Geometry check sheet. Reference: the model listing, model coordinates, mm. A direction names the side the tool comes from. Coordinates: 2 decimals unless noted, no trailing zeros. Loops run counter-clockwise (first coordinate to the right, second up) from the corner with the lowest first, then second, coordinate; pieces in that order, holes last. Notation, with made-up numbers: (0.5, 23) -> (52.5, 23) arc R35 cw to (52.5, 57) -> close; hole circle Ø1 at (50.25, 62). An arc over 180 degrees is marked (long way). Answer as a JSON object with one key per item and string values.
from build123d import *

# Parameters (mm, degrees)
SKETCH_1_R      = 3.5
EXTRUDE_1_DEPTH = 3
FILLET_1_R      = 0.5


with BuildPart() as part:
    # Эскиз1 → Бобышка-Вытянуть1 (new body)
    with BuildSketch(Plane(origin=(0, 0, 0), x_dir=(1, 0, 0), z_dir=(0, 1, 0))):
        Polygon((-56.25, -20.75), (56.25, -20.75), (56.25, -15.25), (59.25, -15.25), (59.25, -5.25), (56.25, -5.25), (56.25, 0), (-56.25, 0), (-56.25, -5.25), (-59.25, -5.25), (-59.25, -15.25), (-56.25, -15.25), align=None)
        with Locations((-40.25, -13.1)):
            Circle(SKETCH_1_R, mode=Mode.SUBTRACT)
        with Locations((-31.305555556, -13.1)):
            Circle(SKETCH_1_R, mode=Mode.SUBTRACT)
        with Locations((-22.361111111, -13.1)):
            Circle(SKETCH_1_R, mode=Mode.SUBTRACT)
        with Locations((-13.416666667, -13.1)):
            Circle(SKETCH_1_R, mode=Mode.SUBTRACT)
        with Locations((-4.472222222, -13.1)):
            Circle(SKETCH_1_R, mode=Mode.SUBTRACT)
        with Locations((4.472222222, -13.1)):
            Circle(SKETCH_1_R, mode=Mode.SUBTRACT)
        with Locations((13.416666667, -13.1)):
            Circle(SKETCH_1_R, mode=Mode.SUBTRACT)
        with Locations((22.361111111, -13.1)):
            Circle(SKETCH_1_R, mode=Mode.SUBTRACT)
        with Locations((31.305555556, -13.1)):
            Circle(SKETCH_1_R, mode=Mode.SUBTRACT)
        with Locations((40.25, -13.1)):
            Circle(SKETCH_1_R, mode=Mode.SUBTRACT)
    extrude(amount=EXTRUDE_1_DEPTH)

    # Скругление1
    fillet_1_edges = [part.edges().sort_by_distance(p)[0] for p in [
        (-59.25, 1.5, 15.25),
        (-59.25, 1.5, 5.25),
        (59.25, 1.5, 5.25),
        (59.25, 1.5, 15.25),
    ]]
    fillet(fillet_1_edges, radius=FILLET_1_R)


solid = part.part
1. Section check B-B, the plane y = 1.8. State how many separate pieces and enclosed holes the cut face has, then the cut area to 3 significant figures.
Evaluation:
{"separate pieces": "1", "enclosed holes": "10", "area": "2,010 mm^2"}
2. Section check A-A, the plane x = 40.25. Record the boundary of the cut face in (y, z), then the cut area to 4 significant figures.
Evaluation:
{"outline": "(0, 0) -> (3, 0) -> (3, 9.6) -> (0, 9.6) -> close; (0, 16.6) -> (3, 16.6) -> (3, 20.75) -> (0, 20.75) -> close", "area": "41.25 mm^2"}
3. Section check D-D, the plane x = 12. Record the boundary of the cut face in (y, z).
Evaluation:
{"outline": "(0, 0) -> (3, 0) -> (3, 9.9) -> (0, 9.9) -> close; (0, 16.3) -> (3, 16.3) -> (3, 20.75) -> (0, 20.75) -> close"}
4. Tool access check on faces 1 (the face through (58, 1, 5.25)), 2 (the face through (56.25, 1, 18)), 3 (the face through (-57, 1, 5.25)), 4 (the face through (-58, 1, 15.25)). Record the directions out of +Z, -Z, +X, -X, +Y, -Y that give a thin tool (end or side, any length) a straight path to the whole face; none if there is none.
Evaluation:
{"face 1": "-Z, +X, +Y, -Y", "face 2": "+Z, +X, +Y, -Y", "face 3": "-Z, -X, +Y, -Y", "face 4": "+Z, -X, +Y, -Y"}
5. Depth check by flat-ended pin: P1, Ø1.5, axis at y = 1.5, z = 4, coming from the +X side; P2, Ø4, axis at x = -13.42, z = 13.1, coming from the +Y side; P3, Ø3, axis at x = 3, z = 9.5, coming from the -Y side; P4, Ø0.8, axis at x = -57, y = 1.5, coming from the +Z side. Enter the tip coordinate at first touch or a pass-through.
Evaluation:
{"P1": "stops at x = 56.25", "P2": "passes through", "P3": "stops at y = 0", "P4": "stops at z = 15.25"}
6. Mould release check, pull along Z, two halves, no side actions. Record for faces 5 (the face through (-1, 1, 20.75)), 6 (the face through (-56.25, 1, 18)), 7 (the face through (27.81, 1.48, 12.95)): released by +Z, released by -Z, zero draft, split by the parting line, or undercut.
Evaluation:
{"face 5": "released by +Z", "face 6": "zero draft", "face 7": "undercut"}
7. Thickness scan on probe 1 along Z at (x, y) = (40.25, 2.1); probe 2 along X at (y, z) = (0.5, 2); probe 3 along Z at (x, y) = (11.5, 0.15). Record the ranges inside material, lowest first. Write a range as from..to.
Evaluation:
{"probe 1": "z = 0..9.6, 16.6..20.75", "probe 2": "x = -56.25..56.25", "probe 3": "z = 0..10.17, 16.03..20.75"}
